from build123d import *

# Parameters (mm, degrees)
SKETCH1_W                   = 53.34
SKETCH1_H                   = 415.925
BOSS_EXTRUDE2_DEPTH         = 6.35
SKETCH2_W                   = 38.1
SKETCH2_H                   = 400.685
CUT_EXTRUDE1_DEPTH          = 448.967600787
F_17_0_173_DIAMETER_HOLE1_D = 4.3942
CUT_EXTRUDE2_DEPTH          = 448.967600787
CUT_EXTRUDE2_DEPTH_BACK     = 448.967600787
SKETCH5_W                   = 2.619375
SKETCH5_H                   = 6.35


with BuildPart() as part:
    # Sketch1 → Boss-Extrude2 (new body)
    with BuildSketch(Plane.XY):
        with Locations((-148.231422107, 204.401588398)):
            Rectangle(SKETCH1_W, SKETCH1_H)
    extrude(amount=BOSS_EXTRUDE2_DEPTH)

    # Sketch2 → Cut-Extrude1 (cut, through all)
    with BuildSketch(Plane(origin=(0, 0, 0), x_dir=(-1, 0, 0), z_dir=(0, 0, -1))):
        with Locations((148.231422107, 204.401588398)):
            Rectangle(SKETCH2_W, SKETCH2_H)
    extrude(amount=-CUT_EXTRUDE1_DEPTH, mode=Mode.SUBTRACT)

    # #17 (0.173) Diameter Hole1 (through all)
    with Locations(Plane(origin=(0, 0, 0), x_dir=(-1, 0, 0), z_dir=(0, 0, -1))):
        with Locations((171.091422107, 408.554088398), (148.231422107, 204.401588398), (171.091422107, 0.249088398), (125.371422107, 408.554088398), (125.371422107, 0.249088398)):
            Hole(F_17_0_173_DIAMETER_HOLE1_D / 2)

    # Sketch5 → Cut-Extrude2 (cut, two sides: drawn at the far end of the back side and taken through both)
    with BuildSketch(Plane.XY.offset(6.35).offset(-CUT_EXTRUDE2_DEPTH_BACK)):
        with Locations((-168.591109607, 394.901588398)):
            Rectangle(SKETCH5_W, SKETCH5_H)
        with Locations((-168.591109607, 13.901588398)):
            Rectangle(SKETCH5_W, SKETCH5_H)
    extrude(amount=CUT_EXTRUDE2_DEPTH + CUT_EXTRUDE2_DEPTH_BACK, mode=Mode.SUBTRACT)


solid = part.part
Source: CAD feature listing. Evaluate the final solid. Frame: model axes, mm. A direction names the side the tool comes from. Round coordinates to 2 decimals unless told otherwise and drop trailing zeros. Write each loop counter-clockwise with the first axis right and the second up, starting at its lowest first coordinate (ties: lowest second). Pieces come first, ordered by that corner, then holes. Notation, with made-up numbers: (-21.75, 23) - (2.25, 23) arc R24 cw to (2.25, 59) - close; hole circle Ø1 at (15.5, 77.5). An arc over 180 degrees is marked (long way). Use CSV: the item, a comma, the result in double quotes. Start each with the question number.
(1) Mould query, pull axis Y, two halves, no side actions, for faces 3 (the face through (-149, 412.364, 3)), 4 (the face through (-129, 221, 6.35)), 5 (the face through (-129.181, 202, 3)). Classes: pulls with the +Y half, pulls with the -Y half, needs draft (parallel to the pull), parting line crosses it, or undercut.
(2) Set-up query: faces 1 (the face through (-174.901, 201, 3)), 2 (the face through (-169.901, 14, 3)). Return all of +Z, -Z, +X, -X, +Y, -Y with unobstructed straight access to the full face (end or side cutting, diameter ignored); none if empty.
(3) Cut plane C-C, the plane z = 2. Return loops of the section in (x, y), and give its area (3 significant figures).
(4) First-contact query: pin 1 Ø7 at (x, y) = (-125.37, 408.55) entering from +Z. Flat tip, straight axial feed; report the tip coordinate or a pass-through.
(5) Cut plane A-A, the plane x = -154. Return loops of the section in (y, z), and give its area (3 significant figures).
(6) Cut plane B-B, the plane y = 208.5. Return loops of the section in (x, z).
(7) Material intervals for probe 1 along Y at (x, z) = (-125, 3.5); probe 2 along Y at (x, z) = (-145.5, 2.75); probe 3 along X at (y, z) = (135, 4.5), sorted ascending. Write a range as [from, to].
Geometry says:
1,face 3,"pulls with the +Y half"
1,face 4,"needs draft"
1,face 5,"undercut"
2,face 1,"+Z, -Z, -X, +Y, -Y"
2,face 2,"+Z, -Z"
3,outline,"(-174.9, -3.56) - (-121.56, -3.56) - (-121.56, 412.36) - (-174.9, 412.36) - close; hole circle Ø4.39 at (-171.09, 0.25); hole circle Ø4.39 at (-171.09, 408.55); hole (-169.9, 10.73) - (-167.28, 10.73) - (-167.28, 4.06) - (-129.18, 4.06) - (-129.18, 404.74) - (-167.28, 404.74) - (-167.28, 398.08) - (-169.9, 398.08) - (-169.9, 391.73) - (-167.28, 391.73) - (-167.28, 17.08) - (-169.9, 17.08) - close; hole circle Ø4.39 at (-125.37, 0.25); hole circle Ø4.39 at (-125.37, 408.55)"
3,area,"6,830 mm²"
4,pin 1,"z = 6.35"
5,outline,"(-3.56, 0) - (4.06, 0) - (4.06, 6.35) - (-3.56, 6.35) - close; (404.74, 0) - (412.36, 0) - (412.36, 6.35) - (404.74, 6.35) - close"
5,area,"96.8 mm²"
6,outline,"(-174.9, 0) - (-167.28, 0) - (-167.28, 6.35) - (-174.9, 6.35) - close; (-129.18, 0) - (-121.56, 0) - (-121.56, 6.35) - (-129.18, 6.35) - close"
7,probe 1,"[-3.56, -1.92], [2.41, 406.39], [410.72, 412.36]"
7,probe 2,"[-3.56, 4.06], [404.74, 412.36]"
7,probe 3,"[-174.9, -167.28], [-129.18, -121.56]"
